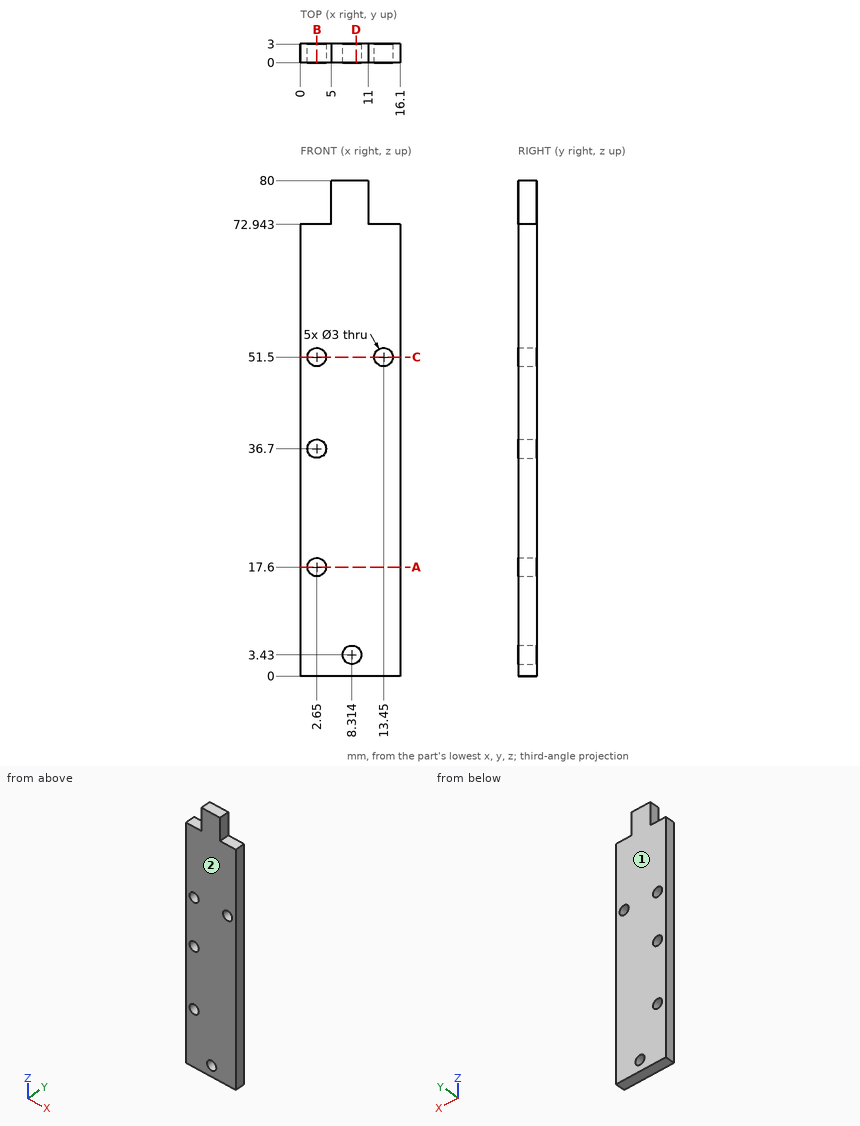
Here's the drawing with two shaded views (mm, measured from the low corner). I have some questions. Give positions to 0.01 mm unless a question says otherwise; leave off trailing zeros. Loops run counter-clockwise (first coordinate to the right, second up) from the corner with the lowest first, then second, coordinate; pieces in that order, holes last. Notation, with made-up numbers: (14, -11.5) - (26, -11.5) arc R32 ccw to (26, 15.5) - close; hole circle Ø6 at (72, 57.25). An arc over 180 degrees is marked (long way). Answer in a Markdown table with one row per item. Add a question column.
Q1. If we section it at D-D (x = 9): List the corners of the cut face in (y, z) for me (1 decimal), plus the area to 3 significant figures.
Q2. If we section it at B-B (x = 2.65): List the corners of the cut face in (y, z) for me, plus the area to 3 significant figures.
Q3. For pin 1 (0.9 mm diameter, centred on y = 2, z = 78, fed in from -X), with a flat end and sliding along its axis, tell me the tip position at first contact or that it passes through.
Q4. We'd pull the mould along Y, two halves only. Please class the marked faces 1 and 2: +Y half, -Y half, draft (parallel to the pull), parting line (faces both ways), or undercut.
Q5. Please list where these lines run through material, in increasing order: L1, parallel to Z at x = 2.65, y = 1.9; L2, parallel to X at y = 1.1, z = 51.5; L3, parallel to Z at x = 13.45, y = 2.1. Write a range as from..to.
Q6. If we section it at C-C (z = 51.5): List the corners of the cut face in (x, y) for me.
Q7. If we section it at A-A (z = 17.6): List the corners of the cut face in (x, y) for me.
The answers:
| question | item | result |
|---|---|---|
| 1 | outline | (0, 0) - (3, 0) - (3, 2.1) - (0, 2.1) - close; (0, 4.8) - (3, 4.8) - (3, 80) - (0, 80) - close |
| 1 | area | 232 mm^2 |
| 2 | outline | (0, 0) - (3, 0) - (3, 16.1) - (0, 16.1) - close; (0, 19.1) - (3, 19.1) - (3, 35.2) - (0, 35.2) - close; (0, 38.2) - (3, 38.2) - (3, 50) - (0, 50) - close; (0, 53) - (3, 53) - (3, 72.94) - (0, 72.94) - close |
| 2 | area | 192 mm^2 |
| 3 | pin 1 | stops at x = 5 |
| 4 | face 1 | +Y half |
| 4 | face 2 | -Y half |
| 5 | L1 | z = 0..16.1, 19.1..35.2, 38.2..50, 53..72.94 |
| 5 | L2 | x = 0..1.15, 4.15..11.95, 14.95..16.1 |
| 5 | L3 | z = 0..50, 53..72.94 |
| 6 | outline | (0, 0) - (1.15, 0) - (1.15, 3) - (0, 3) - close; (4.15, 0) - (11.95, 0) - (11.95, 3) - (4.15, 3) - close; (14.95, 0) - (16.1, 0) - (16.1, 3) - (14.95, 3) - close |
| 7 | outline | (0, 0) - (1.15, 0) - (1.15, 3) - (0, 3) - close; (4.15, 0) - (16.1, 0) - (16.1, 3) - (4.15, 3) - close |
